The model under review builds one solid part; all positions refer to its coordinate system, in mm. A direction names the side the tool comes from. Coordinates: 2 decimals unless noted, no trailing zeros. Order: outer loops, then holes, each group sorted by start corner. A loop starts at its lowest first (then second) coordinate and runs counter-clockwise, first axis right, second up.
```python
from build123d import *

# Parameters (mm, degrees)
BOSS_EXTRUDE1_DEPTH            = 57.15
SKETCH2_R                      = 25.4
CUT_EXTRUDE1_DEPTH             = 57.15
SKETCH3_R                      = 2.2225
CUT_EXTRUDE2_DEPTH             = 57.15
CIRPATTERN1_COUNT              = 4
CUT_EXTRUDE3_REACH             = 120.117
SKETCH4_W                      = 111.76
SKETCH4_H                      = 44.45
CUT_EXTRUDE3_DIRECTION_2_REACH = 120.117
SKETCH5_R                      = 2.2225
CUT_EXTRUDE4_DEPTH             = 6.35


with BuildPart() as part:
    # Sketch1 → Boss-Extrude1 (new body)
    with BuildSketch(Plane(origin=(0, 0, 0), x_dir=(1, 0, 0), z_dir=(0, 1, 0))):
        with BuildLine():
            Line((-39.722823422, 13.362088137), (-69.85, -76.2))
            Line((-69.85, -76.2), (69.85, -76.2))
            Line((69.85, -76.2), (39.722823422, 13.362088137))
            ThreePointArc((39.722823422, 13.362088137), (0, 41.91), (-39.722823422, 13.362088137))
        make_face()
    extrude(amount=BOSS_EXTRUDE1_DEPTH)

    # Sketch2 → Cut-Extrude1 (cut)
    with BuildSketch(Plane(origin=(0, 57.15, 0), x_dir=(1, 0, 0), z_dir=(0, 1, 0))):
        with Locations(Location((0, 0, 0), (0, 0, 270))):
            Circle(SKETCH2_R)
    extrude(amount=-CUT_EXTRUDE1_DEPTH, mode=Mode.SUBTRACT)

    # Sketch3 → Cut-Extrude2 (cut)
    with BuildSketch(Plane(origin=(0, 57.15, 0), x_dir=(1, 0, 0), z_dir=(0, 1, 0))):
        with Locations(Location((0, 38.1, 0), (0, 0, 270))):
            Circle(SKETCH3_R)
    cut_extrude2 = extrude(amount=-CUT_EXTRUDE2_DEPTH, mode=Mode.SUBTRACT)

    # CirPattern1: Cut-Extrude2 ×4 about axis
    cirpattern1_axis = Axis((0, 0, 0), (0, 1, 0))
    for i in range(1, CIRPATTERN1_COUNT):
        add(cut_extrude2.rotate(cirpattern1_axis, i * 360 / CIRPATTERN1_COUNT), mode=Mode.SUBTRACT)

    # Cut-Extrude3: up to this plane
    cut_extrude3_end = Plane(origin=(-39.722823422, 57.15, -13.362088137), z_dir=(0.9478125369142922, 0, 0.318828158838101))
    # Sketch4 → Cut-Extrude3 (cut, up to the surface)
    with BuildSketch(Plane(origin=(0, 0, 0), x_dir=(0, 0, -1), z_dir=(1, 0, 0)), mode=Mode.PRIVATE) as cut_extrude3_sk1:
        with Locations((-13.97, 28.575)):
            Rectangle(SKETCH4_W, SKETCH4_H)
    cut_extrude3_tool1 = split(extrude(cut_extrude3_sk1.sketch, amount=-CUT_EXTRUDE3_REACH, mode=Mode.PRIVATE), bisect_by=cut_extrude3_end, keep=Keep.BOTH, mode=Mode.PRIVATE)
    add(cut_extrude3_tool1.solids().sort_by_distance((0, 28.575, 13.97))[0], mode=Mode.SUBTRACT)

    # Cut-Extrude3 direction 2: up to this plane
    cut_extrude3_direction_2_end = Plane(origin=(39.722823422, 57.15, -13.362088137), z_dir=(0.9478125369142922, 0, -0.318828158838101))
    # Sketch4 → Cut-Extrude3 direction 2 (cut, up to the surface)
    with BuildSketch(Plane(origin=(0, 0, 0), x_dir=(0, 0, -1), z_dir=(1, 0, 0)), mode=Mode.PRIVATE) as cut_extrude3_direction_2_sk1:
        with Locations((-13.97, 28.575)):
            Rectangle(SKETCH4_W, SKETCH4_H)
    cut_extrude3_direction_2_tool1 = split(extrude(cut_extrude3_direction_2_sk1.sketch, amount=CUT_EXTRUDE3_DIRECTION_2_REACH, mode=Mode.PRIVATE), bisect_by=cut_extrude3_direction_2_end, keep=Keep.BOTH, mode=Mode.PRIVATE)
    add(cut_extrude3_direction_2_tool1.solids().sort_by_distance((0, 28.575, 13.97))[0], mode=Mode.SUBTRACT)

    # Sketch5 → Cut-Extrude4 (cut)
    with BuildSketch(Plane.XY.offset(76.2)):
        with Locations((0, 36.5125)):
            Circle(SKETCH5_R)
        with Locations((-7.9375, 28.575)):
            Circle(SKETCH5_R)
        with Locations((0, 20.6375)):
            Circle(SKETCH5_R)
        with Locations((7.9375, 28.575)):
            Circle(SKETCH5_R)
    extrude(amount=-CUT_EXTRUDE4_DEPTH, mode=Mode.SUBTRACT)


solid = part.part
```
(1) Wall thickness on probe 1 along Y at (x, z) = (0, 74.5) (3 decimals); probe 2 along Y at (x, z) = (-31, 7): over which ranges is each line inside the solid? List them lowest first.
A:
probe 1: y = 0 to 18.415, 22.86 to 34.29, 38.735 to 57.15
probe 2: y = 0 to 6.35, 50.8 to 57.15
(2) Machinability: for faces 1 (the face through (-0.29, 22.84, 73.07)), 2 (the face through (1, 50.8, 27)), which of the approach directions +Z, -Z, +X, -X, +Y, -Y give a long, thin tool a straight path to every point of the face, cutting with its end or side? Answer none if there is none.
A:
face 1: +Z, -Z
face 2: -Z, +X, -X
(3) We need section A-A, the plane x = 12. Write out the cut boundary in (y, z), and give its area (3 significant figures).
A:
outline: (0, -40.16) - (6.35, -40.16) - (6.35, -22.39) - (0, -22.39) - close; (0, 22.39) - (6.35, 22.39) - (6.35, 69.85) - (50.8, 69.85) - (50.8, 22.39) - (57.15, 22.39) - (57.15, 76.2) - (0, 76.2) - close; (50.8, -40.16) - (57.15, -40.16) - (57.15, -22.39) - (50.8, -22.39) - close
area: 1,190 mm2
(4) We need section C-C, the plane z = -38.1. Write out the cut boundary in (x, y).
A:
outline: (-17.46, 0) - (-2.22, 0) - (-2.22, 6.35) - (-17.46, 6.35) - close; (-17.46, 50.8) - (-2.22, 50.8) - (-2.22, 57.15) - (-17.46, 57.15) - close; (2.22, 0) - (17.46, 0) - (17.46, 6.35) - (2.22, 6.35) - close; (2.22, 50.8) - (17.46, 50.8) - (17.46, 57.15) - (2.22, 57.15) - close
(5) Draft analysis for pull direction X (two halves, no side actions). For faces 3 (the face through (0.851, 3.219, 36.047)), 4 (the face through (-1, 28, 76.2)), 5 (the face through (0.731, 3.131, -41.904)), 6 (the face through (36.047, 3.219, -0.851)), state which applies: released by +X, released by -X, zero draft, split by the parting line, or undercut.
A:
face 3: undercut
face 4: zero draft
face 5: split by the parting line
face 6: undercut
(6) We need section B-B, the plane z = 0. Count the separate pieces of the cut face and the enclosed holes in it, and give its area (3 significant figures).
A:
separate pieces: 8
enclosed holes: 0
area: 365 mm2
(7) We need section D-D, the plane y = 44. Write out the cut boundary in (x, z).
A:
outline: (-69.85, 76.2) - (-67.71, 69.85) - (67.71, 69.85) - (69.85, 76.2) - close
(8) For pin 1 Ø5 at (y, z) = (8.5, 56.5) entering from +X; pin 2 Ø3 at (x, y) = (-6, 38) entering from -Z, all flat-tipped, find the tip position at first contact; note any pin that passes through.
A:
pin 1: stops at x = 63.65
pin 2: stops at z = 69.85
